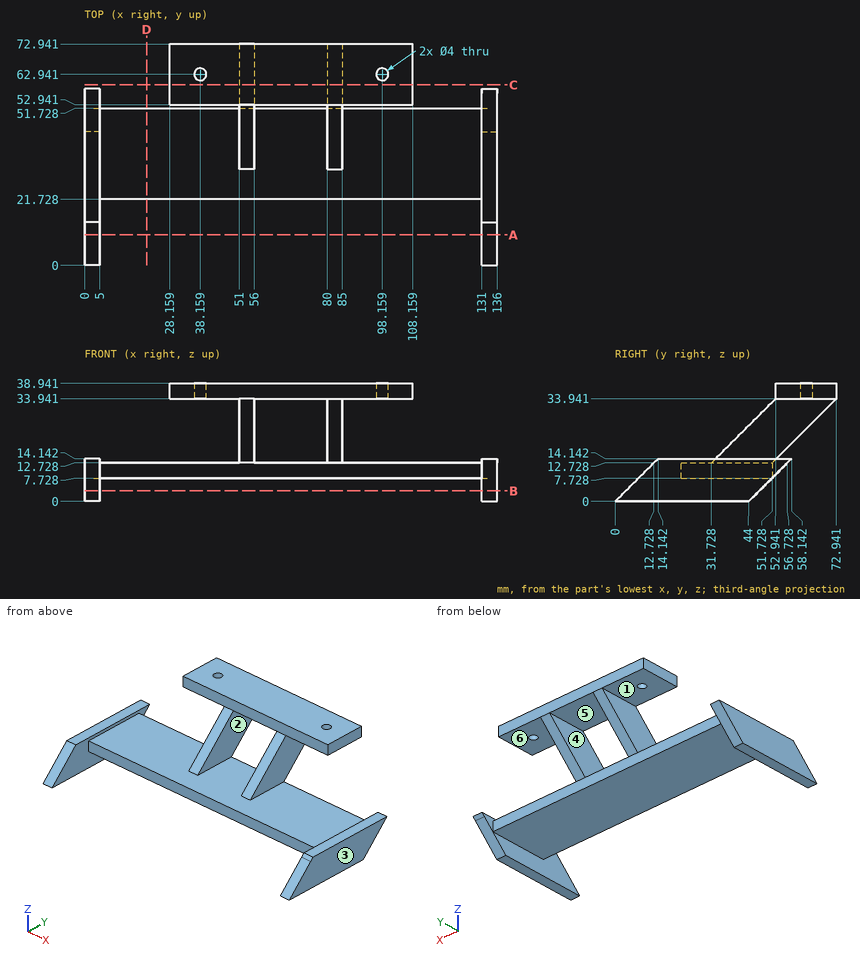
Design review of the part shown in the three views and the two pictorial views. Dimensions are in mm from the part's minimum x, y and z. A direction names the side the tool comes from. Coordinates: 2 decimals unless noted, no trailing zeros. Order: outer loops, then holes, each group sorted by start corner. A loop starts at its lowest first (then second) coordinate and runs counter-clockwise, first axis right, second up.
Item 1: Take a section at A-A, the plane y = 10. Write out the cut boundary in (x, z), then the cut area to 3 significant figures.
Item 2: For pin 1 Ø4 at (y, z) = (18.5, 8) entering from -X; pin 2 Ø6.5 at (y, z) = (54, 25.5) entering from +X; pin 3 Ø6.5 at (x, y) = (98.16, 62.94) entering from -Z; pin 4 Ø12 at (x, y) = (30, 29.5) entering from +Z, all flat-tipped, find the tip position at first contact; note any pin that passes through.
Item 3: The part is to be moulded in two halves that separate along X. For the marked faces 1, 2 and 3, say which applies: pulls with the +X half, pulls with the -X half, needs draft (parallel to the pull), parting line crosses it, or undercut.
Item 4: Take a section at C-C, the plane y = 59.5. Write out the cut boundary in (x, z).
Item 5: For line 1 (Z direction, x = 96, y = 34); line 2 (X direction, y = 21.5, z = 5.5); line 3 (Z direction, x = 40, y = 67), list the stretches that pass through material, from the lowest coordinate up.
Item 6: Take a section at D-D, the plane x = 20.5. Write out the cut boundary in (y, z).
Item 7: Take a section at B-B, the plane z = 3.5. Write out the cut boundary in (x, y), then the cut area to 3 significant figures.
Item 8: For the marked faces 4, 5 and 6, list the 3-axis set-ups (+Z, -Z, +X, -X, +Y, -Y) from which the entire face can be reached by the end or side of a thin tool; tool diameter is ignored.
The answers:
1. outline: (0, 0) - (5, 0) - (5, 10) - (0, 10) - close; (131, 0) - (136, 0) - (136, 10) - (131, 10) - close
1. area: 100 mm2
2. pin 1: stops at x = 0
2. pin 2: stops at x = 85
2. pin 3: stops at z = 33.94
2. pin 4: stops at z = 12.73
3. face 1: needs draft
3. face 2: undercut
3. face 3: pulls with the +X half
4. outline: (28.16, 33.94) - (51, 33.94) - (51, 20.5) - (56, 20.5) - (56, 33.94) - (80, 33.94) - (80, 20.5) - (85, 20.5) - (85, 33.94) - (108.16, 33.94) - (108.16, 38.94) - (28.16, 38.94) - close
5. line 1: z = 7.73 to 12.73
5. line 2: x = 0 to 5, 131 to 136
5. line 3: z = 33.94 to 38.94
6. outline: (21.73, 7.73) - (51.73, 7.73) - (51.73, 12.73) - (21.73, 12.73) - close
7. outline: (0, 3.5) - (5, 3.5) - (5, 47.5) - (0, 47.5) - close; (131, 3.5) - (136, 3.5) - (136, 47.5) - (131, 47.5) - close
7. area: 440 mm2
8. face 4: +Y, -Y
8. face 5: -Z, +Y, -Y
8. face 6: -Z, +X, +Y, -Y
